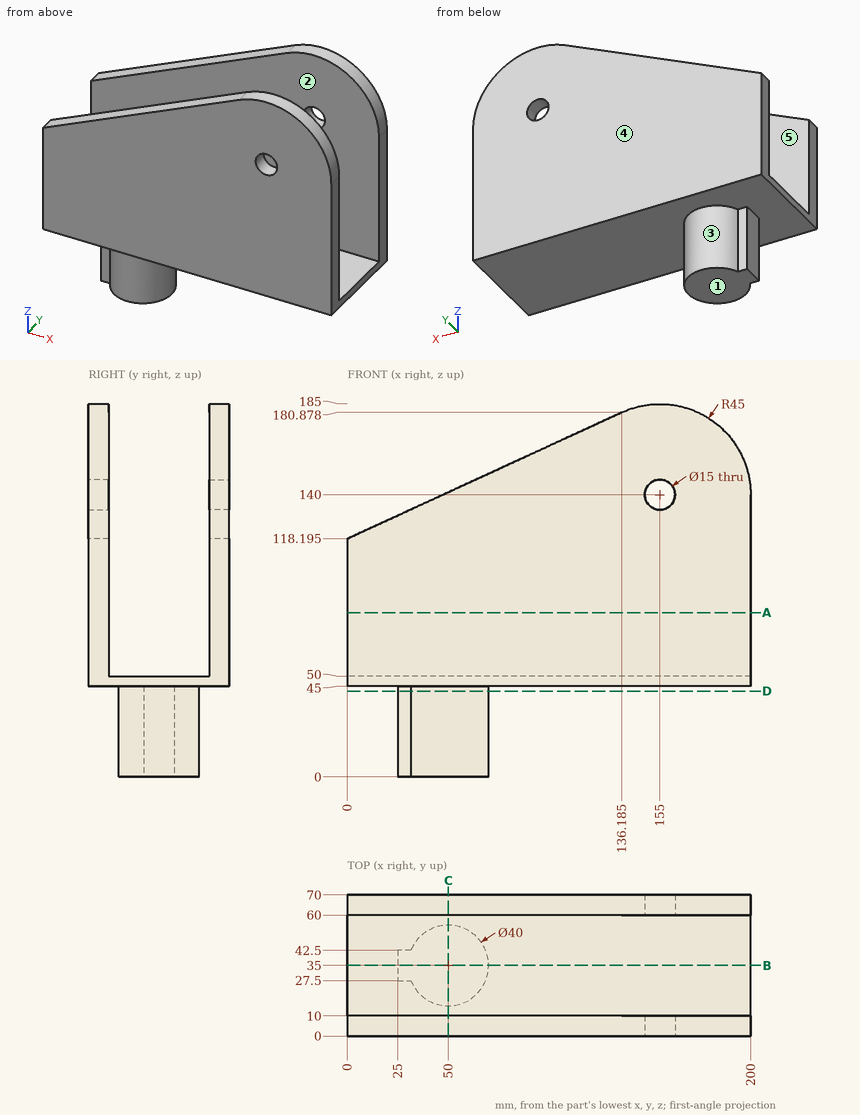
Answer from the drawing. Dimensions are ordinates in mm from the lowest x, y and z of the part. A direction names the side the tool comes from. Give positions to 0.01 mm unless a question says otherwise; leave off trailing zeros. Loops run counter-clockwise (first coordinate to the right, second up) from the corner with the lowest first, then second, coordinate; pieces in that order, holes last. Notation, with made-up numbers: (87.5, 85) - (117.5, 85) arc R18 ccw to (117.5, 109) - close; hole circle Ø11 at (44, 53). An arc over 180 degrees is marked (long way). Answer as CSV lines item,"result". Start each with the question number.
Item 1: For the marked faces 1 and 2, determine the directions among +Z, -Z, +X, -X, +Y, -Y from which every point of the face is accessible in a straight line to the end or side of a thin tool.
Item 2: The mould has two halves that part along Y. Classify the marked faces 3, 4 and 5: +Y half, -Y half, draft (parallel to the pull), parting line (faces both ways), or undercut.
Item 3: Each of these flat-tipped pins is pushed along its axis until it touches: pin 1 (12 mm diameter, centred on y = 35, z = 25.5, fed in from -X); pin 2 (3 mm diameter, centred on x = 27, z = 30, fed in from +Y); pin 3 (12 mm diameter, centred on x = 155, z = 140, fed in from -Y); pin 4 (6 mm diameter, centred on x = 21.5, y = 35, fed in from +Z). Where does it stop, or does it pass through?
Item 4: A cutting plane is placed at B-B on y = 35. Determine the outline of the cut face in (x, z), then the cut area to 4 significant figures.
Item 5: A cutting plane is placed at D-D on z = 42.5. Determine the outline of the cut face in (x, y).
Item 6: A cutting plane is placed at C-C on x = 50. Determine the outline of the cut face in (y, z).
Item 7: Find the intervals of material crossed by line 1 (Y direction, x = 176.5, z = 69); line 2 (Z direction, x = 140, y = 20.5); line 3 (X direction, y = 7.75, z = 140) (1 decimal), in increasing order. Write a range as from..to.
Item 8: A cutting plane is placed at A-A on z = 81.5. Determine the outline of the cut face in (x, y).
Found:
1,face 1,"-Z, +X, -X, +Y, -Y"
1,face 2,"+Z, +X, -X"
2,face 3,"parting line"
2,face 4,"+Y half"
2,face 5,"undercut"
3,pin 1,"stops at x = 25"
3,pin 2,"stops at y = 42.5"
3,pin 3,"passes through"
3,pin 4,"stops at z = 50"
4,outline,"(0, 45) - (25, 45) - (25, 0) - (70, 0) - (70, 45) - (200, 45) - (200, 50) - (0, 50) - close"
4,area,"3,025 mm^2"
5,outline,"(25, 27.5) - (31.46, 27.5) arc R20 ccw (long way) to (31.46, 42.5) - (25, 42.5) - close"
6,outline,"(0, 45) - (15, 45) - (15, 0) - (55, 0) - (55, 45) - (70, 45) - (70, 141.21) - (60, 141.21) - (60, 50) - (10, 50) - (10, 141.21) - (0, 141.21) - close"
7,line 1,"y = 0..10, 60..70"
7,line 2,"z = 45..50"
7,line 3,"x = 47.4..147.5, 162.5..200"
8,outline,"(0, 0) - (200, 0) - (200, 10) - (0, 10) - close; (0, 60) - (200, 60) - (200, 70) - (0, 70) - close"
